```python
from build123d import *

# Parameters (mm, degrees)
SKETCH_3_R      = 2
SKETCH_3_W      = 0.91875
SKETCH_3_H      = 15
SKETCH_3_R_2    = 1.8
EXTRUDE_2_DEPTH = 2


with BuildPart() as part:
    # 草图3 → 凸台-拉伸2 (new body)
    with BuildSketch(Plane(origin=(0, 0, 0), x_dir=(1, 0, 0), z_dir=(0, 1, 0))):
        Polygon((16.9, -21.5), (20.65, -21.5), (20.65, -27), (27, -27), (27, 27), (-4.1, 27), (-4.1, 20), (-16.7, 20), (-16.7, 27), (-27, 27), (-27, -27), (8.65, -27), (8.65, -21.5), (12.4, -21.5), (12.4, -6), (16.9, -6), align=None)
        with Locations((-19.3, 10.3)):
            Circle(SKETCH_3_R, mode=Mode.SUBTRACT)
        with Locations((-2.1, -16.5)):
            Circle(SKETCH_3_R, mode=Mode.SUBTRACT)
        with Locations((-16.4, -3.7)):
            Circle(SKETCH_3_R, mode=Mode.SUBTRACT)
        with Locations((-10.896875, -5.8)):
            Rectangle(SKETCH_3_W, SKETCH_3_H, mode=Mode.SUBTRACT)
        with Locations((-8.140625, -5.8)):
            Rectangle(SKETCH_3_W, SKETCH_3_H, mode=Mode.SUBTRACT)
        with Locations((-5.384375, -5.8)):
            Rectangle(SKETCH_3_W, SKETCH_3_H, mode=Mode.SUBTRACT)
        with Locations((-2.628125, -5.8)):
            Rectangle(SKETCH_3_W, SKETCH_3_H, mode=Mode.SUBTRACT)
        with Locations((0.128125, -5.8)):
            Rectangle(SKETCH_3_W, SKETCH_3_H, mode=Mode.SUBTRACT)
        with Locations((2.884375, -5.8)):
            Rectangle(SKETCH_3_W, SKETCH_3_H, mode=Mode.SUBTRACT)
        with Locations((23.5, -23.5)):
            Circle(SKETCH_3_R_2, mode=Mode.SUBTRACT)
        with Locations((5.640625, -5.8)):
            Rectangle(SKETCH_3_W, SKETCH_3_H, mode=Mode.SUBTRACT)
        with Locations((8.396875, -5.8)):
            Rectangle(SKETCH_3_W, SKETCH_3_H, mode=Mode.SUBTRACT)
        with Locations((-1.1, 15.8)):
            Circle(SKETCH_3_R, mode=Mode.SUBTRACT)
        with Locations((23.5, 23.5)):
            Circle(SKETCH_3_R_2, mode=Mode.SUBTRACT)
        with Locations((-23.5, -23.5)):
            Circle(SKETCH_3_R_2, mode=Mode.SUBTRACT)
        with Locations((-23.5, 23.5)):
            Circle(SKETCH_3_R_2, mode=Mode.SUBTRACT)
    extrude(amount=EXTRUDE_2_DEPTH)


solid = part.part
```
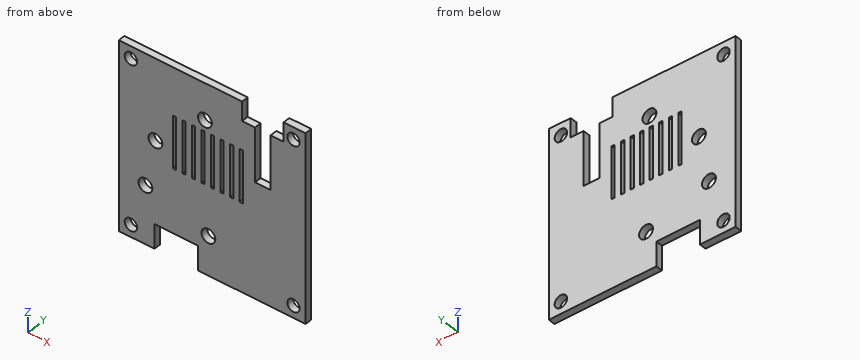
Could you check a few things on this model? Use its own coordinates, in mm. Round coordinates to 2 decimals unless told otherwise and drop trailing zeros. Loops run counter-clockwise (first coordinate to the right, second up) from the corner with the lowest first, then second, coordinate; pieces in that order, holes last. Notation, with made-up numbers: (64.5, 5) -> (123.5, 5) arc R21 ccw to (123.5, 40) -> close; hole circle Ø5 at (-30, 58.5). An arc over 180 degrees is marked (long way). Put each result on its own line as item: value.
Q1. For pin 1 Ø3 at (x, z) = (23.5, 23.5) entering from -Y, with a flat end and sliding along its axis, tell me the tip position at first contact or that it passes through.
Checks:
pin 1: through
Q2. I want a section at B-B on z = -10.3. Write out the boundary of the cut face in (x, y).
Checks:
outline: (-27, 0) -> (-21.3, 0) -> (-21.3, 2) -> (-27, 2) -> close; (-17.3, 0) -> (27, 0) -> (27, 2) -> (-17.3, 2) -> close
Q3. I want a section at C-C on x = -23.5. Write out the boundary of the cut face in (y, z), and give its area (3 significant figures).
Checks:
outline: (0, -27) -> (2, -27) -> (2, -25.3) -> (0, -25.3) -> close; (0, -21.7) -> (2, -21.7) -> (2, 21.7) -> (0, 21.7) -> close; (0, 25.3) -> (2, 25.3) -> (2, 27) -> (0, 27) -> close
area: 93.6 mm2
Q4. Please list where these lines run through material, in increasing order: line 1 (Z direction, x = 23.5, y = 0.3); line 2 (X direction, y = 0.5, z = -23.5); line 3 (X direction, y = 1.8, z = -24). Write a range as from..to.
Checks:
line 1: -27..-25.3, -21.7..21.7, 25.3..27
line 2: -27..-25.3, -21.7..-16.7, -4.1..21.7, 25.3..27
line 3: -27..-25.23, -21.77..-16.7, -4.1..21.77, 25.23..27
Q5. I want a section at A-A on z = -23.5. Write out the boundary of the cut face in (x, y), and give its area (3 significant figures).
Checks:
outline: (-27, 0) -> (-25.3, 0) -> (-25.3, 2) -> (-27, 2) -> close; (-21.7, 0) -> (-16.7, 0) -> (-16.7, 2) -> (-21.7, 2) -> close; (-4.1, 0) -> (21.7, 0) -> (21.7, 2) -> (-4.1, 2) -> close; (25.3, 0) -> (27, 0) -> (27, 2) -> (25.3, 2) -> close
area: 68.4 mm2
Q6. I want a section at D-D on y = 1. Give the number of separate pieces and of enclosed holes in the cut face, and give its area (3 significant figures).
Checks:
separate pieces: 1
enclosed holes: 16
area: 2,490 mm2
